from build123d import *

# Parameters (mm, degrees)
F0_W     = 358.775
F0_H     = 717.55
F1_DEPTH = 19.05
F3_D     = 8.001
F3_DEPTH = 25.4
F3_TIP   = 2.4037429064
F5_D     = 8.001
F5_DEPTH = 25.4
F5_TIP   = 2.4037429064
F7_D     = 15.0114
F7_DEPTH = 14.224
F7_TIP   = 4.5098795482


with BuildPart() as f1:
    # F0 (on Top) → F1 (new body)
    with BuildSketch(Plane.XY):
        Rectangle(F0_W, F0_H)
    extrude(amount=F1_DEPTH)

    # F3
    with Locations(Plane(origin=(-179.3875, 0, 0), x_dir=(0, -1, 0), z_dir=(-1, 0, 0))):
        with Locations((-307.975, 9.525), (0, 9.525), (307.975, 9.525)):
            Hole(F3_D / 2, depth=F3_DEPTH)
            with Locations((0, 0, -(F3_DEPTH + F3_TIP / 2))):  # 118° drill point
                Cone(0, F3_D / 2, F3_TIP, mode=Mode.SUBTRACT)

    # F5
    with Locations(Plane.YZ.offset(179.3875)):
        with Locations((-307.975, 9.525), (0, 9.525), (307.975, 9.525)):
            Hole(F5_D / 2, depth=F5_DEPTH)
            with Locations((0, 0, -(F5_DEPTH + F5_TIP / 2))):  # 118° drill point
                Cone(0, F5_D / 2, F5_TIP, mode=Mode.SUBTRACT)

    # F7
    with Locations(Plane(origin=(0, 0, 0), x_dir=(1, 0, 0), z_dir=(0, 0, -1))):
        with Locations((-155.5115, 307.975), (155.5115, 307.975), (155.5115, 0), (-155.5115, 0), (-155.5115, -307.975), (155.5115, -307.975)):
            Hole(F7_D / 2, depth=F7_DEPTH)
            with Locations((0, 0, -(F7_DEPTH + F7_TIP / 2))):  # 118° drill point
                Cone(0, F7_D / 2, F7_TIP, mode=Mode.SUBTRACT)


solid = f1.part
Verification items for the finished model (mm, model axes). A direction names the side the tool comes from. Coordinates: 2 decimals unless noted, no trailing zeros. One line per item, written item: value. Start each with the question number.
Item 1: Access from +Z, -Z, +X, -X, +Y, -Y to the whole of each face (thin tool, end or side, straight path). Record for faces 1 (the cylindrical face through (-148.013, -308.305, 7.212)), 2 (the flat face through (-3, 358.775, 9)).
Item 2: Mould release check, pull along X, two halves, no side actions. Record for faces 3 (the conical face through (-155.68, -309.27, 17.95)), 4 (the conical face through (156.212, -309.074, 17.951)), 5 (the flat face through (-3, 5, 19.05)), 6 (the flat face through (179.388, -5, 9)): released by +X, released by -X, zero draft, split by the parting line, or undercut.
Item 3: Scan line: probe 1 along Y at (x, z) = (163.5, 10) (3 decimals). Record every from-to range of solid material in increasing order.
Item 4: Gauge pin test, flat ends, axial feed: pin 1 (9 mm diameter, centred on x = -155.51, y = -307.98, fed in from -Z); pin 2 (7 mm diameter, centred on y = 307.975, z = 9.525, fed in from -X). Record the tip position at first contact, or that the pin passes through.
Conclusion:
1. face 1: -Z
1. face 2: +Z, -Z, +X, -X, +Y
2. face 3: undercut
2. face 4: undercut
2. face 5: zero draft
2. face 6: released by +X
3. probe 1: y = -358.775 to -311.947, -304.003 to -3.972, 3.972 to 304.003, 311.947 to 358.775
4. pin 1: stops at z = 16.03
4. pin 2: stops at x = -148.87
